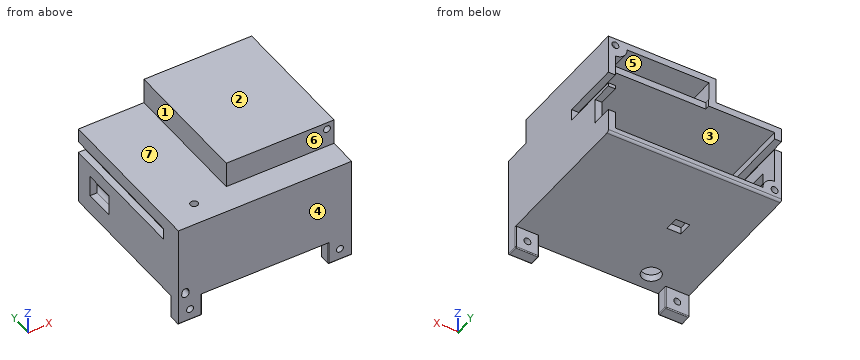
```python
from build123d import *

# Parameters (mm, degrees)
SKETCH1_W            = 74
SKETCH1_H            = 45
BOSS_EXTRUDE1_DEPTH  = 68
SKETCH3_W            = 68
SKETCH3_H            = 39
CUT_EXTRUDE2_DEPTH   = 65
SKETCH13_W           = 68
SKETCH13_H           = 3
BOSS_EXTRUDE3_DEPTH  = 65
SKETCH14_W           = 5
SKETCH14_H           = 58
CUT_EXTRUDE5_DEPTH   = 23
SKETCH15_W           = 5
SKETCH15_H           = 25
CUT_EXTRUDE6_DEPTH   = 3
SKETCH18_R           = 1.6
CUT_EXTRUDE8_DEPTH   = 3
SKETCH20_R           = 4
CUT_EXTRUDE9_DEPTH   = 18
BOSS_EXTRUDE4_DEPTH  = 68
SKETCH23_R           = 1.6
CUT_EXTRUDE10_DEPTH  = 66
BOSS_EXTRUDE5_DEPTH  = 68
SKETCH25_R           = 1.6
CUT_EXTRUDE11_DEPTH  = 66
FILLET2_R            = 1
SKETCH30_W           = 10
SKETCH30_H           = 5
BOSS_EXTRUDE6_DEPTH  = 10
SKETCH33_R           = 1.48
CUT_EXTRUDE13_DEPTH  = 5
SKETCH34_W           = 10
SKETCH34_H           = 5
BOSS_EXTRUDE8_DEPTH  = 10
SKETCH35_R           = 1.48
CUT_EXTRUDE14_DEPTH  = 5
FILLET10_R           = 0.4
CUT_EXTRUDE17_DEPTH  = 11
SKETCH45_W           = 3
SKETCH45_H           = 56
BOSS_EXTRUDE9_DEPTH  = 11
SKETCH47_W           = 46
SKETCH47_H           = 3
BOSS_EXTRUDE10_DEPTH = 11
SKETCH49_R           = 1.48
CUT_EXTRUDE18_DEPTH  = 56
SKETCH50_R           = 1.48
CUT_EXTRUDE19_DEPTH  = 68
SKETCH52_W           = 39.849234896
SKETCH52_H           = 2
CUT_EXTRUDE20_DEPTH  = 3
SKETCH54_W           = 11
SKETCH54_H           = 9
CUT_EXTRUDE21_DEPTH  = 3
SKETCH56_W           = 9
SKETCH56_H           = 13
CUT_EXTRUDE22_DEPTH  = 3
SKETCH57_W           = 6
SKETCH57_H           = 6
CUT_EXTRUDE23_DEPTH  = 3


with BuildPart() as part:
    # Sketch1 → Boss-Extrude1 (new body)
    with BuildSketch(Plane(origin=(-3.580186039, 0, -14.417736579), x_dir=(1, 0, 0), z_dir=(0, 1, 0))):
        with Locations((12.716824493, 5.25)):
            Rectangle(SKETCH1_W, SKETCH1_H)
    extrude(amount=BOSS_EXTRUDE1_DEPTH)

    # Sketch3 → Cut-Extrude2 (cut)
    with BuildSketch(Plane(origin=(-3.580186039, 68, -14.417736579), x_dir=(1, 0, 0), z_dir=(0, 1, 0))):
        with Locations((12.716824493, 5.25)):
            Rectangle(SKETCH3_W, SKETCH3_H)
    extrude(amount=-CUT_EXTRUDE2_DEPTH, mode=Mode.SUBTRACT)

    # Sketch13 → Boss-Extrude3 (add)
    with BuildSketch(Plane(origin=(-3.580186039, 3, -14.417736579), x_dir=(1, 0, 0), z_dir=(0, 1, 0))):
        with Locations((12.716824493, -4.75)):
            Rectangle(SKETCH13_W, SKETCH13_H)
    extrude(amount=BOSS_EXTRUDE3_DEPTH)

    # Sketch14 → Cut-Extrude5 (cut)
    with BuildSketch(Plane(origin=(-27.863361546, 0, -14.417736579), x_dir=(0, 0, 1), z_dir=(-1, 0, 0))):
        with Locations((-2.25, 39)):
            Rectangle(SKETCH14_W, SKETCH14_H)
    extrude(amount=-CUT_EXTRUDE5_DEPTH, mode=Mode.SUBTRACT)

    # Sketch15 → Cut-Extrude6 (cut)
    with BuildSketch(Plane(origin=(46.136638454, 0, -14.417736579), x_dir=(0, 0, -1), z_dir=(1, 0, 0))):
        with Locations((2.25, 55.5)):
            Rectangle(SKETCH15_W, SKETCH15_H)
    extrude(amount=-CUT_EXTRUDE6_DEPTH, mode=Mode.SUBTRACT)

    # Sketch18 → Cut-Extrude8 (cut)
    with BuildSketch(Plane(origin=(-3.580186039, 0, -11.167736579), x_dir=(-1, 0, 0), z_dir=(0, 0, -1))):
        with Locations((11.283175507, 10)):
            Circle(SKETCH18_R)
    extrude(amount=-CUT_EXTRUDE8_DEPTH, mode=Mode.SUBTRACT)

    # Sketch20 → Cut-Extrude9 (cut)
    with BuildSketch(Plane(origin=(0, 0, -42.167736579), x_dir=(-1, 0, 0), z_dir=(0, 0, -1))):
        with Locations((9.863361546, 8)):
            Circle(SKETCH20_R)
    extrude(amount=-CUT_EXTRUDE9_DEPTH, mode=Mode.SUBTRACT)

    # Sketch21 → Boss-Extrude4 (add)
    with BuildSketch(Plane.XZ):
        with BuildLine():
            Line((46.136638454, -4.167736579), (46.136638454, 2.832263421))
            Line((46.136638454, 2.832263421), (39.136638454, 2.832263421))
            ThreePointArc((39.136638454, 2.832263421), (39.601104548, -3.703270485), (46.136638454, -4.167736579))
        make_face()
    extrude(amount=-BOSS_EXTRUDE4_DEPTH)

    # Sketch23 → Cut-Extrude10 (cut)
    with BuildSketch(Plane.XZ):
        with Locations((43.136638454, -0.167736579)):
            Circle(SKETCH23_R)
    extrude(amount=-CUT_EXTRUDE10_DEPTH, mode=Mode.SUBTRACT)

    # Sketch24 → Boss-Extrude5 (add)
    with BuildSketch(Plane.XZ):
        with BuildLine():
            Line((-20.863361546, -42.167736579), (-27.863361546, -42.167736579))
            Line((-27.863361546, -42.167736579), (-27.863361546, -35.167736579))
            ThreePointArc((-27.863361546, -35.167736579), (-21.327827641, -35.632202673), (-20.863361546, -42.167736579))
        make_face()
    extrude(amount=-BOSS_EXTRUDE5_DEPTH)

    # Sketch25 → Cut-Extrude11 (cut)
    with BuildSketch(Plane.XZ):
        with Locations((-24.863361546, -39.167736579)):
            Circle(SKETCH25_R)
    extrude(amount=-CUT_EXTRUDE11_DEPTH, mode=Mode.SUBTRACT)

    # Fillet2
    fillet2_edges = [part.edges().sort_by_distance(p)[0] for p in [
        (9.136638454, 68, -42.167736579),
    ]]
    fillet(fillet2_edges, radius=FILLET2_R)

    # Sketch30 → Boss-Extrude6 (add)
    with BuildSketch(Plane(origin=(0, 0, -42.167736579), x_dir=(-1, 0, 0), z_dir=(0, 0, -1))):
        with Locations((-41.136638454, 2.5)):
            Rectangle(SKETCH30_W, SKETCH30_H)
    extrude(amount=BOSS_EXTRUDE6_DEPTH)

    # Sketch33 → Cut-Extrude13 (cut)
    with BuildSketch(Plane.XZ):
        with Locations((41.136638454, -47.167736579)):
            Circle(SKETCH33_R)
    extrude(amount=-CUT_EXTRUDE13_DEPTH, mode=Mode.SUBTRACT)

    # Sketch34 → Boss-Extrude8 (add)
    with BuildSketch(Plane(origin=(0, 0, -42.167736579), x_dir=(-1, 0, 0), z_dir=(0, 0, -1))):
        with Locations((22.863361546, 2.5)):
            Rectangle(SKETCH34_W, SKETCH34_H)
    extrude(amount=BOSS_EXTRUDE8_DEPTH)

    # Sketch35 → Cut-Extrude14 (cut)
    with BuildSketch(Plane.XZ):
        with Locations((-22.863361546, -47.167736579)):
            Circle(SKETCH35_R)
    extrude(amount=-CUT_EXTRUDE14_DEPTH, mode=Mode.SUBTRACT)

    # Fillet10
    fillet10_edges = [part.edges().sort_by_distance(p)[0] for p in [
        (46.136638454, 5, -47.167736579),
        (36.136638454, 0, -47.167736579),
        (36.136638454, 5, -47.167736579),
        (46.136638454, 2.5, -52.167736579),
        (41.136638454, 0, -52.167736579),
        (36.136638454, 2.5, -52.167736579),
        (41.136638454, 5, -52.167736579),
        (-17.863361546, 5, -47.167736579),
        (-17.863361546, 0, -47.167736579),
        (-17.863361546, 2.5, -52.167736579),
        (-22.863361546, 0, -52.167736579),
        (-22.863361546, 5, -52.167736579),
    ]]
    fillet(fillet10_edges, radius=FILLET10_R)

    # Sketch43 → Cut-Extrude17 (cut)
    with BuildSketch(Plane.XY.offset(2.832263421)):
        Polygon((-27.863361546, 68), (0.136638454, 68), (0.136638454, 12), (46.136638454, 12), (46.136638454, 0), (-27.863361546, 0), (-27.863361546, 12), align=None)
    extrude(amount=-CUT_EXTRUDE17_DEPTH, mode=Mode.SUBTRACT)

    # Sketch45 → Boss-Extrude9 (add)
    with BuildSketch(Plane.XY.offset(2.832263421)):
        with Locations((1.636638454, 40)):
            Rectangle(SKETCH45_W, SKETCH45_H)
    extrude(amount=-BOSS_EXTRUDE9_DEPTH)

    # Sketch47 → Boss-Extrude10 (add)
    with BuildSketch(Plane.XY.offset(2.832263421)):
        with Locations((23.136638454, 13.5)):
            Rectangle(SKETCH47_W, SKETCH47_H)
    extrude(amount=-BOSS_EXTRUDE10_DEPTH)

    # Sketch49 → Cut-Extrude18 (cut)
    with BuildSketch(Plane(origin=(0, 68, 0), x_dir=(1, 0, 0), z_dir=(0, 1, 0))):
        with Locations((43.136638454, 0.167736579)):
            Circle(SKETCH49_R)
    extrude(amount=-CUT_EXTRUDE18_DEPTH, mode=Mode.SUBTRACT)

    # Sketch50 → Cut-Extrude19 (cut)
    with BuildSketch(Plane(origin=(0, 68, 0), x_dir=(1, 0, 0), z_dir=(0, 1, 0))):
        with Locations((-24.863361546, 38.167736579)):
            Circle(SKETCH50_R)
    extrude(amount=-CUT_EXTRUDE19_DEPTH, mode=Mode.SUBTRACT)

    # Sketch52 → Cut-Extrude20 (cut)
    with BuildSketch(Plane(origin=(0, 0, -11.167736579), x_dir=(-1, 0, 0), z_dir=(0, 0, -1))):
        with Locations((-23.212021006, 67)):
            Rectangle(SKETCH52_W, SKETCH52_H)
    extrude(amount=-CUT_EXTRUDE20_DEPTH, mode=Mode.SUBTRACT)

    # Sketch54 → Cut-Extrude21 (cut)
    with BuildSketch(Plane(origin=(46.136638454, 0, 0), x_dir=(0, 0, -1), z_dir=(1, 0, 0))):
        with Locations((26.2154696, 63.5)):
            Rectangle(SKETCH54_W, SKETCH54_H)
    extrude(amount=-CUT_EXTRUDE21_DEPTH, mode=Mode.SUBTRACT)

    # Sketch56 → Cut-Extrude22 (cut)
    with BuildSketch(Plane.ZY.offset(27.863361546)):
        with Locations((-29.387336529, 53.5)):
            Rectangle(SKETCH56_W, SKETCH56_H)
    extrude(amount=-CUT_EXTRUDE22_DEPTH, mode=Mode.SUBTRACT)

    # Sketch57 → Cut-Extrude23 (cut)
    with BuildSketch(Plane(origin=(0, 0, -42.167736579), x_dir=(-1, 0, 0), z_dir=(0, 0, -1))):
        with Locations((3.863361546, 36)):
            Rectangle(SKETCH57_W, SKETCH57_H)
    extrude(amount=-CUT_EXTRUDE23_DEPTH, mode=Mode.SUBTRACT)


solid = part.part
```
The model under review builds one solid part; all positions refer to its coordinate system, in mm. Face numbers are marked on the shaded views. A direction names the side the tool comes from. Coordinates: 2 decimals unless noted, no trailing zeros. Write each loop counter-clockwise with the first axis right and the second up, starting at its lowest first coordinate (ties: lowest second). Pieces come first, ordered by that corner, then holes.
1) Clearance check with flat-ended pins moving along their axes: pin 1 Ø12 at (x, z) = (7.5, -12) entering from +Y; pin 2 Ø2 at (x, z) = (-9, -32) entering from +Y; pin 3 Ø17.5 at (x, y) = (27.5, 42) entering from -Z; pin 4 Ø1.9 at (x, z) = (43.14, -0.17) entering from -Y. State where each tip first meets the part, or that it passes through.
2) We need section D-D on y = 51. Count the separate pieces of the cut face and the enclosed holes in it, then the cut area to 3 significant figures.
3) To check wall thickness, follow probe 1 along Z at (x, y) = (19, 14.5); probe 2 along Z at (x, y) = (-8.5, 27); probe 3 along Z at (x, y) = (21, 26). State the ranges of each line that lie inside material, in increasing order.
4) We need section C-C on x = 8.5. State the section outline as (y, z) points.
5) We need section B-B on y = 34.5. State the section outline as (x, z) points, then the cut area to 3 significant figures.
6) We need section A-A on z = -29. State the section outline as (x, y) points, then the cut area to 3 significant figures.
7) Machinability: for the marked faces 4, 5, 6 and 7, which of the approach directions +Z, -Z, +X, -X, +Y, -Y give a long, thin tool a straight path to every point of the face, cutting with its end or side? Answer none if there is none.
8) The part is to be moulded in two halves that separate along X. For the marked faces 1, 2 and 3, say which applies: pulls with the +X half, pulls with the -X half, needs draft (parallel to the pull), parting line crosses it, or undercut.
Answer list:
1. pin 1: stops at y = 68
1. pin 2: stops at y = 3
1. pin 3: stops at z = -42.17
1. pin 4: passes through
2. separate pieces: 3
2. enclosed holes: 3
2. area: 762 mm2
3. probe 1: z = -42.17 to -39.17, -11.17 to 2.83
3. probe 2: z = -42.17 to -39.17, -11.17 to -8.17
3. probe 3: z = -42.17 to -39.17, -11.17 to -8.17, -0.17 to 2.83
4. outline: (0, -42.17) - (67, -42.17) arc R1 ccw to (68, -41.17) - (68, -39.17) - (3, -39.17) - (3, -11.17) - (66, -11.17) - (66, -8.17) - (15, -8.17) - (15, -0.17) - (68, -0.17) - (68, 2.83) - (12, 2.83) - (12, -8.17) - (0, -8.17) - close
5. outline: (-27.86, -42.17) - (-6.86, -42.17) - (-6.86, -39.17) - (-19.86, -39.17) arc R5 ccw to (-24.86, -34.17) - (-24.86, -19.17) - (-27.86, -19.17) - close; (-27.86, -14.17) - (-24.86, -14.17) - (-24.86, -11.17) - (43.14, -11.17) - (43.14, -39.17) - (-0.86, -39.17) - (-0.86, -42.17) - (46.14, -42.17) - (46.14, 2.83) - (0.14, 2.83) - (0.14, -8.17) - (-27.86, -8.17) - close; hole (-26.31, -38.48) arc R1.6 ccw (long way) to (-23.42, -38.48) arc R1.48 ccw (long way) to start; hole (3.14, -8.17) - (43.14, -8.17) - (43.14, -5.17) arc R5 cw to (38.14, -0.17) - (3.14, -0.17) - close; hole circle Ø3.2 at (43.14, -0.17)
5. area: 786 mm2
6. outline: (-27.86, 0) - (46.14, 0) - (46.14, 59) - (43.14, 59) - (43.14, 3) - (-24.86, 3) - (-24.86, 47) - (-27.86, 47) - close; (-27.86, 60) - (-24.86, 60) - (-24.86, 68) - (-27.86, 68) - close
6. area: 546 mm2
7. face 4: +Z, -Z, +X, -X, -Y
7. face 5: +Y
7. face 6: +Z, +X, -X, -Y
7. face 7: +Z, -X, -Y
8. face 1: pulls with the -X half
8. face 2: needs draft
8. face 3: undercut
